Model file for the job. Use its own axes, mm. A direction names the side the tool comes from. Coordinates: 2 decimals unless noted, no trailing zeros. Order: outer loops, then holes, each group sorted by start corner. A loop starts at its lowest first (then second) coordinate and runs counter-clockwise, first axis right, second up. Notation, with made-up numbers: (-18.5, 60) -> (-13.5, 60) arc R16 ccw to (-13.5, 83) -> close; hole circle Ø3 at (46.5, 10.5). An arc over 180 degrees is marked (long way). Write item = value, one per line. Start each with the question number.
Q1. Wall check: line 1 (Z direction, x = 976, y = 1); line 2 (Z direction, x = 1650, y = -47.35). Give the ranges that are in metal, low to high. Write a range as from..to.
Q2. Cut at A-A, the plane y = 19. List the corners of the cut face in (x, z), plus the area to 3 significant figures.
Q3. Flat gauge pin, fed straight in: pin 1 (12 mm diameter, centred on y = -37.5, z = 11.5, fed in from +X). Where does the tip first touch, or does it go through?
Q4. 3-axis set-ups, long thin cutter, end or side, ignore diameter. For faces 4 (the face through (838, -1, -50)), 5 (the face through (838, -1, 45)): which of +Z, -Z, +X, -X, +Y, -Y reach the whole face in a straight line?
Q5. Cut at B-B, the plane x = 333. List the corners of the cut face in (y, z), plus the area to 3 significant figures.
Q6. Mould opens along Y. For faces 1 (the face through (1669.076, -47.465, 6.007)), 2 (the face through (838, 50, -1)), 3 (the face through (838, -1, -45)) say: +Y half, -Y half, draft (parallel to the pull), parting line (faces both ways), or undercut.
Q7. Cut at C-C, the plane z = 0. Give the number of separate pieces and of enclosed holes in the cut face, plus the area to 3 significant figures.
from build123d import *

# Parameters (mm, degrees)
F0_W     = 100
F0_H     = 100
F0_W_2   = 90
F0_H_2   = 90
F1_DEPTH = 1700
F2_R     = 20
F3_DEPTH = 50


with BuildPart() as f1:
    # F0 (on Right) → F1 (new body)
    with BuildSketch(Plane.YZ):
        Rectangle(F0_W, F0_H)
        Rectangle(F0_W_2, F0_H_2, mode=Mode.SUBTRACT)
    extrude(amount=F1_DEPTH)

    # F2 (on Front) → F3 (cut, symmetric)
    with BuildSketch(Plane.XZ):
        with Locations((50, 0)):
            Circle(F2_R)
        with Locations((1650, 0)):
            Circle(F2_R)
        with Locations((280, 0)):
            Circle(F2_R)
        with Locations((1420, 0)):
            Circle(F2_R)
    extrude(amount=F3_DEPTH, both=True, mode=Mode.SUBTRACT)


solid = f1.part
Here are the results:
q1.line_1 = -50..-45, 45..50
q1.line_2 = -50..-20, 20..50
q2.outline = (0, -50) -> (1700, -50) -> (1700, -45) -> (0, -45) -> close; (0, 45) -> (1700, 45) -> (1700, 50) -> (0, 50) -> close
q2.area = 17,000 mm²
q3.pin_1 = through
q4.face_4 = -Z, +X, -X, +Y, -Y
q4.face_5 = +X, -X
q5.outline = (-50, -50) -> (50, -50) -> (50, 50) -> (-50, 50) -> close; hole (-45, -45) -> (45, -45) -> (45, 45) -> (-45, 45) -> close
q5.area = 1,900 mm²
q6.face_1 = draft
q6.face_2 = +Y half
q6.face_3 = undercut
q7.separate_pieces = 10
q7.enclosed_holes = 0
q7.area = 15,400 mm²
